For this review, take the finished solid that the model builds, in its own axes (mm). A direction names the side the tool comes from. Coordinates: 2 decimals unless noted, no trailing zeros. Loops run counter-clockwise (first coordinate to the right, second up) from the corner with the lowest first, then second, coordinate; pieces in that order, holes last. Notation, with made-up numbers: M 49.25,-38.75 L 98.25,-38.75 A18 cw 98.25,-34.75 Z; hole C 74.5,35.25 d7. An arc over 180 degrees is marked long. Use one line per item in the form item = value.
```python
from build123d import *

# Parameters (mm, degrees)
SKETCH1_R           = 6.3
BOSS_EXTRUDE1_DEPTH = 5
SKETCH2_R           = 7.5
BOSS_EXTRUDE2_DEPTH = 1.8
SKETCH3_R           = 6
BOSS_EXTRUDE3_DEPTH = 9
SKETCH4_R           = 4.5
CUT_EXTRUDE1_DEPTH  = 10
BOSS_EXTRUDE4_DEPTH = 10
SKETCH6_R           = 0.5
BOSS_EXTRUDE5_DEPTH = 8
FILLET1_R           = 0.2
SKETCH7_R           = 0.75
BOSS_EXTRUDE6_DEPTH = 5
SKETCH8_W           = 10
SKETCH8_H           = 0.5
SKETCH8_H_2         = 1.079785018
CUT_EXTRUDE2_DEPTH  = 5


with BuildPart() as part:
    # Sketch1 → Boss-Extrude1 (new body)
    with BuildSketch(Plane(origin=(0, 0, 0), x_dir=(1, 0, 0), z_dir=(0, 1, 0))):
        Circle(SKETCH1_R)
    extrude(amount=BOSS_EXTRUDE1_DEPTH)

    # Sketch2 → Boss-Extrude2 (add)
    with BuildSketch(Plane(origin=(0, 5, 0), x_dir=(1, 0, 0), z_dir=(0, 1, 0))):
        Circle(SKETCH2_R)
    extrude(amount=BOSS_EXTRUDE2_DEPTH)

    # Sketch3 → Boss-Extrude3 (add)
    with BuildSketch(Plane(origin=(0, 6.8, 0), x_dir=(1, 0, 0), z_dir=(0, 1, 0))):
        Circle(SKETCH3_R)
    extrude(amount=BOSS_EXTRUDE3_DEPTH)

    # Sketch4 → Cut-Extrude1 (cut)
    with BuildSketch(Plane.XZ):
        Circle(SKETCH4_R)
    extrude(amount=-CUT_EXTRUDE1_DEPTH, mode=Mode.SUBTRACT)

    # Sketch5 → Boss-Extrude4 (add)
    with BuildSketch(Plane.XZ.offset(-10)):
        with BuildLine():
            Line((-0.5, 4.5), (0.5, 4.5))
            ThreePointArc((0.5, 4.5), (0, 4), (-0.5, 4.5))
        make_face()
    extrude(amount=BOSS_EXTRUDE4_DEPTH)

    # Sketch6 → Boss-Extrude5 (add)
    with BuildSketch(Plane.XZ.offset(-10)):
        with Locations((-2, 2)):
            Circle(SKETCH6_R)
        with Locations((2, 2)):
            Circle(SKETCH6_R)
        with Locations((2, -2)):
            Circle(SKETCH6_R)
        with Locations((-2, -2)):
            Circle(SKETCH6_R)
    extrude(amount=BOSS_EXTRUDE5_DEPTH)

    # Fillet1
    fillet1_edges = [part.edges().sort_by_distance(p)[0] for p in [
        (-2.5, 2, 2),
        (1.5, 2, 2),
        (1.5, 2, -2),
        (-2.5, 2, -2),
    ]]
    fillet(fillet1_edges, radius=FILLET1_R)

    # Sketch7 → Boss-Extrude6 (add)
    with BuildSketch(Plane(origin=(0, 15.8, 0), x_dir=(1, 0, 0), z_dir=(0, 1, 0))):
        with Locations((-3.138015201, 2.5)):
            Circle(SKETCH7_R)
        with Locations((-3.138015201, -2.5)):
            Circle(SKETCH7_R)
        with Locations((3.015436482, -2.5)):
            Circle(SKETCH7_R)
        with Locations((3.015436482, 2.5)):
            Circle(SKETCH7_R)
    extrude(amount=BOSS_EXTRUDE6_DEPTH)

    # Sketch8 → Cut-Extrude2 (cut)
    with BuildSketch(Plane.XZ):
        with Locations((0, 6.3)):
            Rectangle(SKETCH8_W, SKETCH8_H)
        with Locations((0, -6.3)):
            Rectangle(SKETCH8_W, SKETCH8_H_2)
    extrude(amount=-CUT_EXTRUDE2_DEPTH, mode=Mode.SUBTRACT)


solid = part.part
```
1. Wall thickness on line 1 along X through (y, z) = (2.5, 0); line 2 along Y through (x, z) = (1.75, 3); line 3 along Y through (x, z) = (6, 3.5): over which ranges is each line inside the solid? List them lowest first. Write a range as from..to.
Computed values:
line_1 = -6.3..-4.5, 4.5..6.3
line_2 = 10..15.8
line_3 = 5..6.8
2. Tool access review of faces 4 (the face through (0, 2, 6.05)), 5 (the face through (-0.191, 4.93, -4.496)), 6 (the face through (3.73, 18.26, 2.27)), 7 (the face through (6.278, 2.465, 0.53)): name each direction out of +Z, -Z, +X, -X, +Y, -Y from which nothing blocks a thin tool from reaching the whole face with its end or side.
Computed values:
face_4 = +Z, +X, -X, -Y
face_5 = -Y
face_6 = +Y
face_7 = +X, -Y
3. Draft analysis for pull direction Z (two halves, no side actions). For faces 1 (the face through (1.5, 6.2, -2)), 2 (the face through (-6, 11, 0)), 3 (the face through (0, 5, -6)), state which applies: +Z half, -Z half, draft (parallel to the pull), parting line (faces both ways), or undercut.
Computed values:
face_1 = undercut
face_2 = parting line
face_3 = draft
4. Consider section A-A on y = 7.5. Write out the cut boundary in (x, z).
Computed values:
outline = C 0,0 d12; C -2,-2 d1; C -2,2 d1; C 2,-2 d1; C 2,2 d1; hole M -0.5,4.47 A4.5 ccw long 0.5,4.47 A0.5 cw Z
5. Consider section D-D on z = 5.5. Write out the cut boundary in (x, y).
Computed values:
outline = M -5.1,5 L -3.07,5 L -3.07,0 L 3.07,0 L 3.07,5 L 5.1,5 L 5.1,6.8 L 2.4,6.8 L 2.4,15.8 L -2.4,15.8 L -2.4,6.8 L -5.1,6.8 Z
6. Consider section C-C on x = -3.5. Write out the cut boundary in (y, z), plus the area to 3 significant figures.
Computed values:
outline = M 0,-5.24 L 5,-5.24 L 5,-6.63 L 6.8,-6.63 L 6.8,-4.87 L 15.8,-4.87 L 15.8,-3.16 L 20.8,-3.16 L 20.8,-1.84 L 15.8,-1.84 L 15.8,1.84 L 20.8,1.84 L 20.8,3.16 L 15.8,3.16 L 15.8,4.87 L 6.8,4.87 L 6.8,6.63 L 5,6.63 L 5,5.24 L 0,5.24 L 0,2.83 L 10,2.83 L 10,-2.83 L 0,-2.83 Z
area = 121 mm2
7. Consider section B-B on y = 5.25. Write out the cut boundary in (x, z).
Computed values:
outline = C 0,0 d15; C -2,-2 d1; C -2,2 d1; C 2,-2 d1; C 2,2 d1; hole M -0.5,4.47 A4.5 ccw long 0.5,4.47 A0.5 cw Z
8. For pin 1 Ø0.5 at (x, z) = (2, 2) entering from -Y; pin 2 Ø2.5 at (x, y) = (1, 2) entering from -Z; pin 3 Ø4 at (x, y) = (-4.5, 3.5) entering from -Z, all flat-tipped, find the tip position at first contact; note any pin that passes through.
Computed values:
pin_1 = 2
pin_2 = -5.76
pin_3 = -6.79
